Build history of the part. All positions in model axes, mm. Face numbers are marked on the shaded views. Round coordinates to 2 decimals unless told otherwise and drop trailing zeros. Write each loop counter-clockwise with the first axis right and the second up, starting at its lowest first coordinate (ties: lowest second). Pieces come first, ordered by that corner, then holes.
1) Wall check: probe 1 along Y at (x, z) = (0, 33); probe 2 along X at (y, z) = (0, 26); probe 3 along Y at (x, z) = (-1.5, 30). Give the ranges that are in metal, low to high.
2) Flat gauge pins, fed straight in: pin 1 (0.9 mm diameter, centred on x = 3.5, z = 28, fed in from +Y); pin 2 (1 mm diameter, centred on y = 3, z = 12.5, fed in from -X); pin 3 (2 mm diameter, centred on x = 3.5, y = 1, fed in from +Z); pin 4 (5 mm diameter, centred on x = 4.5, y = 0.5, fed in from -Z). Where does each tip first touch, or does it go through?
3) Pull direction X, two halves, no side cores. Call the marked faces 1, 2 and 3: +X half, -X half, draft (parallel to the pull), parting line (faces both ways), or undercut.
4) Saw through at B-B (z = 14). Write the cut outline in (x, y), plus the area to 3 significant figures.
5) Saw through at A-A (z = 37.5). Write the cut outline in (x, y).
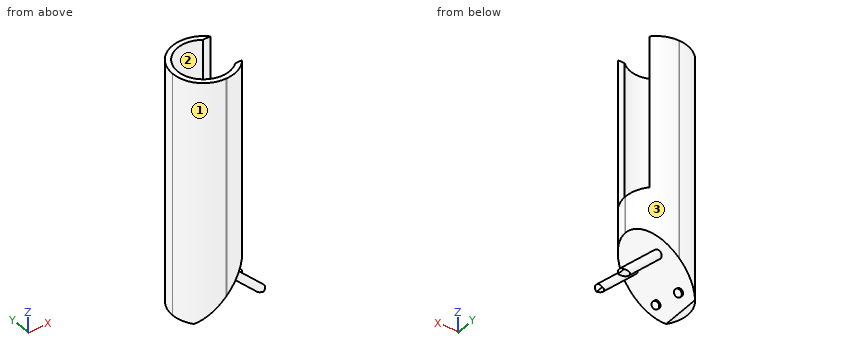
from build123d import *

# Parameters (mm, degrees)
F0_W      = 10.1233841851
F0_H      = 10.0899571553
F1_DEPTH  = 40
F3_D      = 8.5
F3_DEPTH  = 25
F3_TIP    = 2.5536576309
F4_SIZE   = 9
F5_R      = 0.6119078038
F5_R_2    = 0.6255064778
F5_R_3    = 0.6950065758
F5_R_4    = 0.6250316631
F6_DEPTH  = 0.3
F8_DEPTH  = 25
F9_R      = 5
F10_DEPTH = 7.8
F11_W     = 25.9334780276
F11_H     = 20.5789422616
F12_DEPTH = 25


with BuildPart() as f1:
    # F0 (on Top) → F1 (new body)
    with BuildSketch(Plane.XY):
        Rectangle(F0_W, F0_H)
    extrude(amount=F1_DEPTH)

    # F3
    with Locations(Plane.XY.offset(40)):
        with Locations((0, 0)):
            Hole(F3_D / 2, depth=F3_DEPTH)
            with Locations((0, 0, -(F3_DEPTH + F3_TIP / 2))):  # 118° drill point
                Cone(0, F3_D / 2, F3_TIP, mode=Mode.SUBTRACT)

    # F4
    f4_edges = [f1.edges().sort_by_distance(p)[0] for p in [
        (5.061692, 0, 0),
    ]]
    chamfer(f4_edges, length=F4_SIZE)

    # F5 (on face) → F6 (join)
    with BuildSketch(Plane(origin=(-1.9691539537, 0, 1.9691539537), x_dir=(0, 1, 0), z_dir=(0.7071067812, 0, -0.7071067812))):
        with Locations((-2.6314246934, 0)):
            Circle(F5_R)
        with Locations((1.7054068157, -0.6661886582)):
            Circle(F5_R_2)
        with Locations((2.3579068948, 5.0519071519)):
            Circle(F5_R_3)
        with Locations((-2.431909088, 5.4562026635)):
            Circle(F5_R_4)
    extrude(amount=F6_DEPTH)

    # F7 (on face) → F8 (cut)
    with BuildSketch(Plane.XY.offset(40)):
        with BuildLine():
            Line((2.8953096145, -3.1112187702), (5.0616920926, -3.1112187702))
            Line((5.0616920926, -3.1112187702), (5.0616920926, 3.4764062685))
            Line((5.0616920926, 3.4764062685), (2.44481072, 3.4764062685))
            ThreePointArc((2.44481072, 3.4764062685), (3.7717996739, 1.9585778565), (4.25, 0))
            ThreePointArc((4.25, 0), (3.8966373876, -1.6966782456), (2.8953096145, -3.1112187702))
        make_face()
        with BuildLine():
            Line((2.44481072, -3.1112187702), (2.8953096145, -3.1112187702))
            ThreePointArc((2.8953096145, -3.1112187702), (3.8966373876, -1.6966782456), (4.25, 0))
            ThreePointArc((4.25, 0), (3.7717996739, 1.9585778565), (2.44481072, 3.4764062685))
            Line((2.44481072, 3.4764062685), (2.44481072, -3.1112187702))
        make_face()
    extrude(amount=-F8_DEPTH, mode=Mode.SUBTRACT)

    # F9
    f9_edges = [f1.edges().sort_by_distance(p)[0] for p in [
        (-5.061692, 5.044979, 20),
        (-5.061692, -5.044979, 20),
        (5.061692, -5.044979, 24.5),
        (5.061692, 5.044979, 24.5),
    ]]
    fillet(f9_edges, radius=F9_R)

    # F10 (add): faces of the model
    f10_faces = [f1.faces().sort_by_distance(p)[0] for p in [
        (1.8152158857, 2.3579068948, 5.3292597244),
        (2.1010959835, -2.431909088, 5.6151398222),
    ]]
    extrude(f10_faces, amount=F10_DEPTH)

    # F11 (on face) → F12 (cut)
    with BuildSketch(Plane(origin=(0, 0, 0), x_dir=(1, 0, 0), z_dir=(0, 0, -1))):
        with Locations((1.6984669492, -1.4439118095)):
            Rectangle(F11_W, F11_H)
        with BuildLine():
            Line((-3.9383079074, 3.2028021674), (-3.9383079074, -3.2028021674))
            ThreePointArc((-3.9383079074, -3.2028021674), (-4.7724817862, -1.7208247707), (-5.0616920926, -0.0449785776))
            Line((-5.0616920926, -0.0449785776), (-5.0616920926, 0.0449785776))
            ThreePointArc((-5.0616920926, 0.0449785776), (-4.7724817862, 1.7208247707), (-3.9383079074, 3.2028021674))
        make_face(mode=Mode.SUBTRACT)
    extrude(amount=F12_DEPTH, mode=Mode.SUBTRACT)


solid = f1.part
Evaluation:
1. probe 1: y = -5.04 to -4.25, 4.25 to 5.04
1. probe 2: x = -5.06 to -4.25
1. probe 3: y = -4.83 to -3.98, 3.98 to 4.83
2. pin 1: stops at y = 4.05
2. pin 2: stops at x = -4.42
2. pin 3: stops at z = 15
2. pin 4: stops at z = 0
3. face 1: -X half
3. face 2: undercut
3. face 3: +X half
4. outline: (-5.06, -0.04) arc R5 ccw to (-0.06, -5.04) - (0.06, -5.04) arc R5 ccw to (5.06, -0.04) - (5.06, 0.04) arc R5 ccw to (0.06, 5.04) - (-0.06, 5.04) arc R5 ccw to (-5.06, 0.04) - close; hole circle Ø5.17 at (0, 0)
4. area: 59.7 mm2
5. outline: (-5.06, -0.04) arc R5 ccw to (-0.06, -5.04) - (0.06, -5.04) arc R5 ccw to (4.01, -3.11) - (2.9, -3.11) arc R4.25 cw (long way) to (2.44, 3.48) - (3.7, 3.48) arc R5 ccw to (0.06, 5.04) - (-0.06, 5.04) arc R5 ccw to (-5.06, 0.04) - close
